Input: part model. Units: mm. Frame: model coordinates. A direction names the side the tool comes from. Round coordinates to 2 decimals unless told otherwise and drop trailing zeros. Write each loop counter-clockwise with the first axis right and the second up, starting at its lowest first coordinate (ties: lowest second). Pieces come first, ordered by that corner, then holes. Notation, with made-up numbers: M 34,63 L 67,63 A14 ccw 67,85 Z; hole C 74,19 d9. An arc over 180 degrees is marked long. Use one line per item in the form item = value. Start each with the question number.
```python
from build123d import *

# Parameters (mm, degrees)
SKETCH1_R           = 4.572
BOSS_EXTRUDE1_DEPTH = 3.175
SKETCH2_W           = 57.15
SKETCH2_H           = 3.175
BOSS_EXTRUDE2_DEPTH = 2.2098
BOSS_EXTRUDE3_DEPTH = 28.575
BOSS_EXTRUDE4_DEPTH = 57.15


with BuildPart() as part:
    # Sketch1 → Boss-Extrude1 (new body)
    with BuildSketch(Plane.XY):
        with BuildLine():
            Line((59.436, -6.35), (-59.436, -6.35))
            ThreePointArc((-59.436, -6.35), (-63.028102448, -4.862102448), (-64.516, -1.27))
            Line((-64.516, -1.27), (-64.516, 1.27))
            ThreePointArc((-64.516, 1.27), (-63.028102448, 4.862102448), (-59.436, 6.35))
            Line((-59.436, 6.35), (59.436, 6.35))
            ThreePointArc((59.436, 6.35), (63.028102448, 4.862102448), (64.516, 1.27))
            Line((64.516, 1.27), (64.516, -1.27))
            ThreePointArc((64.516, -1.27), (63.028102448, -4.862102448), (59.436, -6.35))
        make_face()
        with Locations((-58.166, 0)):
            Circle(SKETCH1_R, mode=Mode.SUBTRACT)
        with Locations(Location((58.166, 0, 0), (0, 0, 180))):
            Circle(SKETCH1_R, mode=Mode.SUBTRACT)
    extrude(amount=BOSS_EXTRUDE1_DEPTH)

    # Sketch2 → Boss-Extrude2 (add)
    with BuildSketch(Plane.XZ.offset(6.35)):
        with Locations((0, 1.5875)):
            Rectangle(SKETCH2_W, SKETCH2_H)
    boss_extrude2 = extrude(amount=BOSS_EXTRUDE2_DEPTH)

    # Sketch3 → Boss-Extrude3 (add, symmetric)
    with BuildSketch(Plane(origin=(0, 0, 0), x_dir=(0, 0, -1), z_dir=(1, 0, 0))):
        Polygon((-3.175, -8.5598), (-12.2174, -8.5598), (-12.2174, -6.0198), (-6.985, -6.0198), (-6.985, 0.3302), (-3.175, 0.3302), align=None)
    boss_extrude3 = extrude(amount=BOSS_EXTRUDE3_DEPTH, both=True)

    # Mirror1: Boss-Extrude2, Boss-Extrude3 across plane
    add(boss_extrude2.mirror(Plane.ZX))
    add(boss_extrude3.mirror(Plane.ZX))

    # Sketch7 → Boss-Extrude4 (add)
    with BuildSketch(Plane.ZY.offset(28.575)):
        Polygon((12.2174, 8.5598), (4.5974, 14.8082), (4.5974, 8.5598), align=None)
    extrude(amount=-BOSS_EXTRUDE4_DEPTH)


solid = part.part
```
Item 1: Cut plane B-B (z = 2). Output: boundary loops of the cut face in (x, y) (3 decimals).
Item 2: First-contact query: pin 1 (3.5 mm diameter, centred on x = 38, z = 1, fed in from -Y); pin 2 (3.5 mm diameter, centred on x = -2, y = -2.5, fed in from +Z) (3 decimals); pin 3 (1.6 mm diameter, centred on x = 13.5, z = 10, fed in from +Y); pin 4 (3 mm diameter, centred on x = 31, z = 5, fed in from +Y). Flat tips, straight axial feed; report the tip coordinate or a pass-through.
Item 3: Ray query, line 1 (Z direction, x = -40, y = -2.75) (3 decimals); line 2 (Y direction, x = 15.5, z = 8.25); line 3 (Y direction, x = 4, z = 11). Return the intervals inside material, ascending. Write a range as from..to.
Item 4: Cut plane D-D (y = 12.5). Output: boundary loops of the cut face in (x, z) (3 decimals).
Item 5: Cut plane A-A (y = 0). Output: boundary loops of the cut face in (x, z) (3 decimals).
Item 6: Draft query along Y for faces 1 (the face through (-53.943, -1.751, 1.565)), 2 (the face through (0, 8.56, 2)), 3 (the face through (-62.99, -4.9, 1.57)). Return one class per face: +Y half, -Y half, draft (parallel to the pull), parting line (faces both ways), or undercut.
Item 7: Reachability of faces 4 (the face through (0, 6.02, 10)), 5 (the face through (0, 12, 4.597)), 6 (the face through (-44, 6.35, 2)), 7 (the face through (-44, -6.35, 2)), 8 (the face through (44, 6.35, 2)) from +Z, -Z, +X, -X, +Y, -Y: full face, straight path, thin tool, end or side. Return the list, or none.
Item 8: Cut plane C-C (z = 11). Output: boundary loops of the cut face in (x, y) (3 decimals), plus the area to 3 significant figures.
Final values:
q1.outline = M -64.516,-1.27 A5.08 ccw -59.436,-6.35 L -28.575,-6.35 L -28.575,-8.56 L 28.575,-8.56 L 28.575,-6.35 L 59.436,-6.35 A5.08 ccw 64.516,-1.27 L 64.516,1.27 A5.08 ccw 59.436,6.35 L 28.575,6.35 L 28.575,8.56 L -28.575,8.56 L -28.575,6.35 L -59.436,6.35 A5.08 ccw -64.516,1.27 Z; hole C -58.166,0 d9.144; hole C 58.166,0 d9.144
q2.pin_1 = -6.35
q2.pin_2 = 6.985
q2.pin_3 = 11.03
q2.pin_4 = through
q3.line_1 = 0..3.175
q3.line_2 = -8.56..-6.02, 6.02..11.81
q3.line_3 = -8.56..-6.02, 6.02..9.56
q4.outline = M -28.575,4.597 L 28.575,4.597 L 28.575,7.412 L -28.575,7.412 Z
q5.outline = M -64.516,0 L -62.738,0 L -62.738,3.175 L -64.516,3.175 Z; M -53.594,0 L 53.594,0 L 53.594,3.175 L 28.575,3.175 L 28.575,6.985 L -28.575,6.985 L -28.575,3.175 L -53.594,3.175 Z; M 62.738,0 L 64.516,0 L 64.516,3.175 L 62.738,3.175 Z
q6.face_1 = undercut
q6.face_2 = +Y half
q6.face_3 = -Y half
q7.face_4 = +Z, +X, -X
q7.face_5 = -Z, +X, -X, +Y
q7.face_6 = +Z, -Z, -X, +Y
q7.face_7 = +Z, -Z, -X, -Y
q7.face_8 = +Z, -Z, +X, +Y
q8.outline = M -28.575,-8.56 L 28.575,-8.56 L 28.575,-6.02 L -28.575,-6.02 Z; M -28.575,6.02 L 28.575,6.02 L 28.575,9.558 L -28.575,9.558 Z
q8.area = 347 mm^2
